Design review of the part built by this model. Coordinates are the model's own, in mm. Face numbers are marked on the shaded views. Coordinates: 2 decimals unless noted, no trailing zeros. Loops run counter-clockwise (first coordinate to the right, second up) from the corner with the lowest first, then second, coordinate; pieces in that order, holes last. Notation, with made-up numbers: (6, -15) -> (23, -15) arc R26 ccw to (23, 2) -> close; hole circle Ø10 at (88.25, 12). An arc over 180 degrees is marked (long way). Answer as a JSON object with one key per item and string values.
```python
from build123d import *

# Parameters (mm, degrees)
SKICA1_W                 = 68
SKICA1_H                 = 45
SKICA1_R                 = 1.5
SKICA1_R_2               = 5
SKICA1_R_3               = 2.5
P_IDAT_VYSUNUT_M1_DEPTH  = 2.5
SKICA2_W                 = 5
SKICA2_H                 = 5
SKICA2_R                 = 1.5
P_IDAT_VYSUNUT_M2_DEPTH  = 4
ODEBRAT_START            = -2.5
SKICA5_R                 = 1.5
ODEBRAT_VYSUNUT_M1_DEPTH = 2.5
ZKOSEN_1_SIZE            = 1.5


with BuildPart() as part:
    # Skica1 → Přidat vysunutím1 (new body)
    with BuildSketch(Plane.XY):
        Rectangle(SKICA1_W, SKICA1_H)
        with Locations((-31.5, 20)):
            Circle(SKICA1_R, mode=Mode.SUBTRACT)
        with Locations((31.5, 20)):
            Circle(SKICA1_R, mode=Mode.SUBTRACT)
        with Locations((31.5, -20)):
            Circle(SKICA1_R, mode=Mode.SUBTRACT)
        with Locations((-31.5, -20)):
            Circle(SKICA1_R, mode=Mode.SUBTRACT)
        with Locations((-14, 0)):
            Circle(SKICA1_R_2, mode=Mode.SUBTRACT)
        with Locations((14, 0)):
            Circle(SKICA1_R_3, mode=Mode.SUBTRACT)
    extrude(amount=P_IDAT_VYSUNUT_M1_DEPTH)

    # Skica2 → Přidat vysunutím2 (add)
    # profile 1 of 4: a face of its own
    with BuildSketch(Plane.XY.offset(2.5)):
        with Locations((-29.5, 15.5)):
            Rectangle(SKICA2_W, SKICA2_H)
        with Locations((-29.5, 15.5)):
            Circle(SKICA2_R, mode=Mode.SUBTRACT)
    # profile 2 of 4: a face of its own
    with BuildSketch(Plane.XY.offset(2.5)):
        with Locations((1.5, 15.5)):
            Rectangle(SKICA2_W, SKICA2_H)
        with Locations((1.5, 15.5)):
            Circle(SKICA2_R, mode=Mode.SUBTRACT)
    # profile 3 of 4: a face of its own
    with BuildSketch(Plane.XY.offset(2.5)):
        with Locations((1.5, -15.5)):
            Rectangle(SKICA2_W, SKICA2_H)
        with Locations((1.5, -15.5)):
            Circle(SKICA2_R, mode=Mode.SUBTRACT)
    # profile 4 of 4: a face of its own
    with BuildSketch(Plane.XY.offset(2.5)):
        with Locations((-29.5, -15.5)):
            Rectangle(SKICA2_W, SKICA2_H)
        with Locations((-29.5, -15.5)):
            Circle(SKICA2_R, mode=Mode.SUBTRACT)
    extrude(amount=P_IDAT_VYSUNUT_M2_DEPTH)

    # Skica5 → Odebrat vysunutím1 (cut)
    with BuildSketch(Plane.XY.offset(2.5).offset(ODEBRAT_START)):
        with Locations((-29.5, 15.5)):
            Circle(SKICA5_R)
        with Locations((1.5, 15.5)):
            Circle(SKICA5_R)
        with Locations((1.5, -15.5)):
            Circle(SKICA5_R)
        with Locations((-29.5, -15.5)):
            Circle(SKICA5_R)
    extrude(amount=ODEBRAT_VYSUNUT_M1_DEPTH, mode=Mode.SUBTRACT)

    # Zkosení1
    zkosen_1_edges = [part.edges().sort_by_distance(p)[0] for p in [
        (0, -15.5, 0),
        (0, 15.5, 0),
        (-31, 15.5, 0),
        (-31, -15.5, 0),
    ]]
    chamfer(zkosen_1_edges, length=ZKOSEN_1_SIZE)


solid = part.part
```
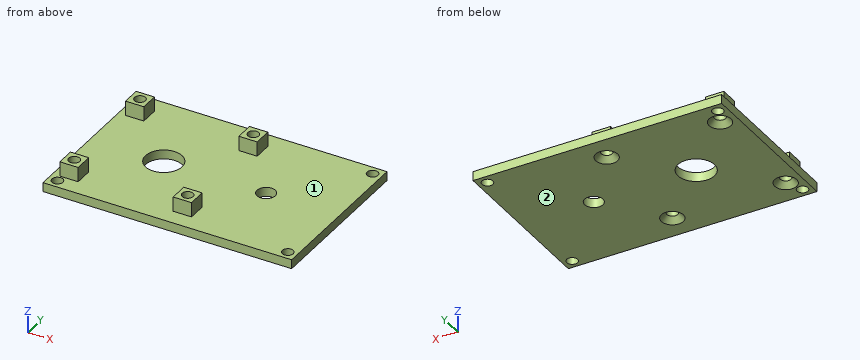
1) Wall thickness on probe 1 along Y at (x, z) = (31.5, 1.6); probe 2 along Y at (x, z) = (-29.5, 4.4); probe 3 along X at (y, z) = (1, 0.5): over which ranges is each line inside the solid? List them lowest first.
Completed:
{"probe 1": "-22.5 to -21.5, -18.5 to 18.5, 21.5 to 22.5", "probe 2": "-18 to -17, -14 to -13, 13 to 14, 17 to 18", "probe 3": "-34 to -18.9, -9.1 to 11.71, 16.29 to 34"}
2) The part is to be moulded in two halves that separate along Y. For the marked faces 1 and 2, say which applies: pulls with the +Y half, pulls with the -Y half, needs draft (parallel to the pull), parting line crosses it, or undercut.
Completed:
{"face 1": "undercut", "face 2": "needs draft"}
3) Add section A-A, the plane x = 14. Give the boundary of the cut face in (y, z), and give its area (3 significant figures).
Completed:
{"outline": "(-22.5, 0) -> (-2.5, 0) -> (-2.5, 2.5) -> (-22.5, 2.5) -> close; (2.5, 0) -> (22.5, 0) -> (22.5, 2.5) -> (2.5, 2.5) -> close", "area": "100 mm²"}
4) Add section B-B, the plane z = 5.5. Give the boundary of the cut face in (x, y), and give its area (3 significant figures).
Completed:
{"outline": "(-32, -18) -> (-27, -18) -> (-27, -13) -> (-32, -13) -> close; (-32, 13) -> (-27, 13) -> (-27, 18) -> (-32, 18) -> close; (-1, -18) -> (4, -18) -> (4, -13) -> (-1, -13) -> close; (-1, 13) -> (4, 13) -> (4, 18) -> (-1, 18) -> close; hole circle Ø3 at (-29.5, -15.5); hole circle Ø3 at (-29.5, 15.5); hole circle Ø3 at (1.5, -15.5); hole circle Ø3 at (1.5, 15.5)", "area": "71.7 mm²"}
5) Clearance check with flat-ended pins moving along their axes: pin 1 Ø2 at (y, z) = (-14.5, 4) entering from -X; pin 2 Ø3 at (x, z) = (-29, 5) entering from +Y; pin 3 Ø3 at (x, z) = (-29, 5) entering from -Y. State where each tip first meets the part, or that it passes through.
Completed:
{"pin 1": "x = -32", "pin 2": "y = 18", "pin 3": "y = -18"}
6) Add section D-D, the plane x = 1.5. Give the boundary of the cut face in (y, z).
Completed:
{"outline": "(-22.5, 0) -> (-18.5, 0) -> (-17, 1.5) -> (-17, 6.5) -> (-18, 6.5) -> (-18, 2.5) -> (-22.5, 2.5) -> close; (-14, 1.5) -> (-12.5, 0) -> (12.5, 0) -> (14, 1.5) -> (14, 6.5) -> (13, 6.5) -> (13, 2.5) -> (-13, 2.5) -> (-13, 6.5) -> (-14, 6.5) -> close; (17, 1.5) -> (18.5, 0) -> (22.5, 0) -> (22.5, 2.5) -> (18, 2.5) -> (18, 6.5) -> (17, 6.5) -> close"}
7) Add section C-C, the plane y = 15.5. Give the boundary of the cut face in (x, z), and give its area (4 significant figures).
Completed:
{"outline": "(-34, 0) -> (-32.5, 0) -> (-31, 1.5) -> (-31, 6.5) -> (-32, 6.5) -> (-32, 2.5) -> (-34, 2.5) -> close; (-28, 1.5) -> (-26.5, 0) -> (-1.5, 0) -> (0, 1.5) -> (0, 6.5) -> (-1, 6.5) -> (-1, 2.5) -> (-27, 2.5) -> (-27, 6.5) -> (-28, 6.5) -> close; (3, 1.5) -> (4.5, 0) -> (34, 0) -> (34, 2.5) -> (4, 2.5) -> (4, 6.5) -> (3, 6.5) -> close", "area": "166.5 mm²"}
